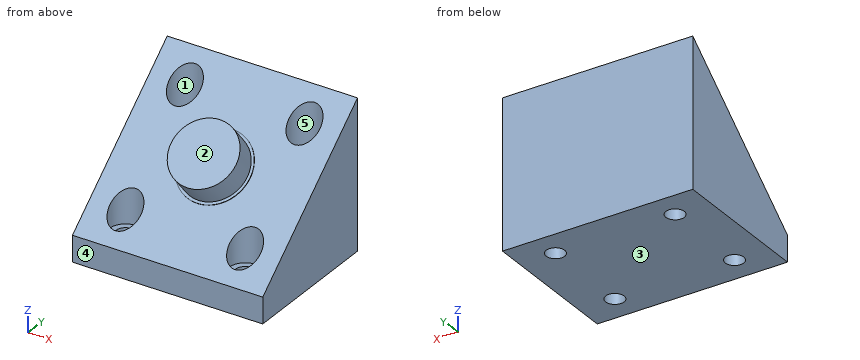
from build123d import *

# Parameters (mm, degrees)
AUFSATZ_LINEAR_AUSTRAGEN1_DEPTH      = 35
SKIZZE3_R                            = 6
AUFSATZ_LINEAR_AUSTRAGEN2_DEPTH      = 5
SKIZZE4_R                            = 6.5
AUFSATZ_LINEAR_AUSTRAGEN3_DEPTH      = 0.1
SKIZZE7_R                            = 2.85
SCHNITT_LINEAR_AUSTRAGEN1_DEPTH      = 23.497566339
F_3_4_3_4_DURCHMESSER_BOHRUNG1_D     = 3.4
F_3_4_3_4_DURCHMESSER_BOHRUNG1_DEPTH = 4.79
K_RPER_VERSCHIEBEN_KOPIEREN1_ANGLE   = 90


with BuildPart() as part:
    # Skizze1 → Aufsatz-Linear austragen1 (new body)
    with BuildSketch(Plane(origin=(0, 0, 0), x_dir=(0, 0, -1), z_dir=(1, 0, 0))):
        Polygon((0, 0), (26.811555509, 0), (26.811555509, 27.287566339), (0, 4.79), align=None)
    extrude(amount=AUFSATZ_LINEAR_AUSTRAGEN1_DEPTH)

    # Skizze3 → Aufsatz-Linear austragen2 (add)
    with BuildSketch(Plane(origin=(0, 2.810887386, 2.358614568), x_dir=(1, 0, 0), z_dir=(0, 0.766044443, 0.64278761))):
        with Locations((17.5, 20.57895265)):
            Circle(SKIZZE3_R)
    extrude(amount=AUFSATZ_LINEAR_AUSTRAGEN2_DEPTH)

    # Skizze4 → Aufsatz-Linear austragen3 (add)
    with BuildSketch(Plane(origin=(0, 2.810887386, 2.358614568), x_dir=(1, 0, 0), z_dir=(0, 0.766044443, 0.64278761))):
        with Locations((17.5, 20.57895265)):
            Circle(SKIZZE4_R)
    extrude(amount=AUFSATZ_LINEAR_AUSTRAGEN3_DEPTH)

    # Skizze7 → Schnitt-Linear austragen1 (cut, through all)
    with BuildSketch(Plane(origin=(0, 4.79, 0), x_dir=(-1, 0, 0), z_dir=(0, -1, 0))):
        with Locations((-28.5, 21.811555509)):
            Circle(SKIZZE7_R)
        with Locations((-6.5, 21.811555509)):
            Circle(SKIZZE7_R)
        with Locations((-6.5, 5)):
            Circle(SKIZZE7_R)
        with Locations((-28.5, 5)):
            Circle(SKIZZE7_R)
    extrude(amount=-SCHNITT_LINEAR_AUSTRAGEN1_DEPTH, mode=Mode.SUBTRACT)

    # Ø3.4 (3.4) Durchmesser Bohrung1
    with Locations(Plane(origin=(6.5, 4.79, -21.811555509), x_dir=(0, 0, 1), z_dir=(0, 1, 0))):
        with Locations((0, 0), (16.811555509, 0), (16.811555509, 22), (0, 22)):
            Hole(F_3_4_3_4_DURCHMESSER_BOHRUNG1_D / 2, depth=F_3_4_3_4_DURCHMESSER_BOHRUNG1_DEPTH)


with BuildPart() as part_1:
    # Körper-Verschieben/Kopieren1: moved
    add(part.part.rotate(Axis((0, 13.64378317, -13.405777755), (1, 0, 0)), K_RPER_VERSCHIEBEN_KOPIEREN1_ANGLE))


solid = part_1.part
Part model, mm, in its own coordinate system. Face numbers are marked on the shaded views. A direction names the side the tool comes from. Coordinates: 2 decimals unless noted, no trailing zeros. Loops run counter-clockwise (first coordinate to the right, second up) from the corner with the lowest first, then second, coordinate; pieces in that order, holes last. Notation, with made-up numbers: (-32.5, -31.75) -> (4.5, -31.75) arc R20 cw to (4.5, -2.75) -> close; hole circle Ø9 at (-9.75, 30.25). An arc over 180 degrees is marked (long way). Use a Markdown table: item, result. Add a question column.
Item 1: Band-saw the part on D-D on x = 3. Write the cut outline in (y, z), plus the area to 3 significant figures.
Item 2: Band-saw the part on B-B on x = 6.5. Write the cut outline in (y, z).
Item 3: Pull direction Y, two halves, no side cores. Call the marked faces 3, 4 and 5: +Y half, -Y half, draft (parallel to the pull), parting line (faces both ways), or undercut.
Item 4: Which spindle directions (+Z, -Z, +X, -X, +Y, -Y) get a long thin tool onto all of the face, cutting with end or side? Do the marked faces 1 and 2. Say none if no direction does.
Item 5: Band-saw the part on C-C on z = -17. Write the cut outline in (x, y), plus the area to 3 significant figures.
Item 6: Band-saw the part on A-A on z = -23.5. Write the cut outline in (x, y).
Item 7: Probe probe 1 along Y at (x, z) = (6.5, -17.75); probe 2 along X at (y, z) = (20.25, -14); probe 3 along Z at (x, y) = (22, 9.5). List the from-to ranges inside material, lowest first.
Item 8: Flat gauge pins, fed straight in: P1, Ø5, axis at y = 22, z = -6, coming from the -X side; P2, Ø3, axis at x = 28.5, y = 5.24, coming from the -Z side; P3, Ø4.5, axis at x = 6.5, y = 22.05, coming from the +Z side; P4, Ø4, axis at x = 9, y = 24, coming from the +Z side. Where does each tip first touch, or does it go through?
Geometry says:
| question | item | result |
|---|---|---|
| 1 | outline | (0.24, -27.05) -> (27.05, -27.05) -> (27.05, 0.24) -> (0.24, -22.26) -> close |
| 1 | area | 430 mm² |
| 2 | outline | (0.24, -27.05) -> (3.54, -27.05) -> (3.54, -22.26) -> (2.39, -22.26) -> (2.39, -20.46) -> (0.24, -22.26) -> close; (6.94, -27.05) -> (20.35, -27.05) -> (20.35, -22.26) -> (19.2, -22.26) -> (19.2, -6.35) -> (8.09, -15.67) -> (8.09, -22.26) -> (6.94, -22.26) -> close; (23.75, -27.05) -> (27.05, -27.05) -> (27.05, 0.24) -> (24.9, -1.57) -> (24.9, -22.26) -> (23.75, -22.26) -> close |
| 3 | face 3 | draft |
| 3 | face 4 | -Y half |
| 3 | face 5 | undercut |
| 4 | face 1 | +Z |
| 4 | face 2 | +Z, +X, -X, -Y |
| 5 | outline | (0, 6.51) -> (3.95, 6.51) arc R2.85 cw to (9.05, 6.51) -> (25.95, 6.51) arc R2.85 cw to (31.05, 6.51) -> (35, 6.51) -> (35, 27.05) -> (0, 27.05) -> close; hole circle Ø5.7 at (6.5, 22.05); hole circle Ø5.7 at (28.5, 22.05) |
| 5 | area | 656 mm² |
| 6 | outline | (0, 0.24) -> (35, 0.24) -> (35, 27.05) -> (0, 27.05) -> close; hole circle Ø3.4 at (6.5, 5.24); hole circle Ø3.4 at (6.5, 22.05); hole circle Ø3.4 at (28.5, 5.24); hole circle Ø3.4 at (28.5, 22.05) |
| 7 | probe 1 | 8.09 to 19.2, 24.9 to 27.05 |
| 7 | probe 2 | 0 to 4.29, 8.71 to 26.29, 30.71 to 35 |
| 7 | probe 3 | -27.05 to -14.49, -12.25 to -7.96 |
| 8 | P1 | x = 0 |
| 8 | P2 | through |
| 8 | P3 | z = -22.26 |
| 8 | P4 | z = -0.64 |
